For this review, take the finished solid that the model builds, in its own axes (mm). Give positions to 0.01 mm unless a question says otherwise; leave off trailing zeros. Write each loop counter-clockwise with the first axis right and the second up, starting at its lowest first coordinate (ties: lowest second). Pieces come first, ordered by that corner, then holes. Notation, with made-up numbers: (-25.75, 76) -> (-17.75, 76) arc R33 cw to (-17.75, 110) -> close; hole circle Ø8 at (86.5, 26.25). An arc over 180 degrees is marked (long way). Return JSON: item names as keys, results as strings.
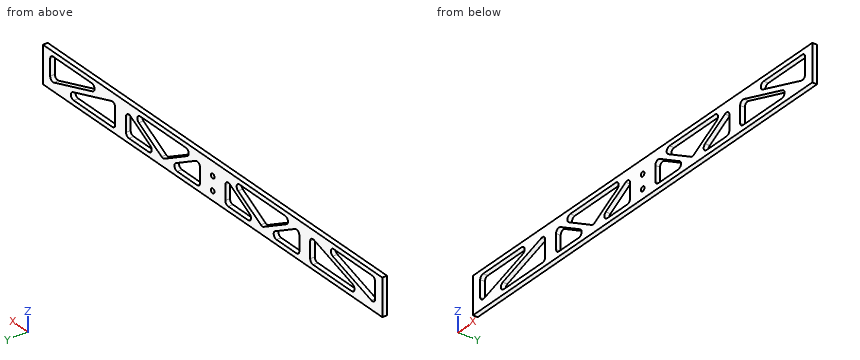
from build123d import *

# Parameters (mm, degrees)
SKETCH1_W           = 298.45
SKETCH1_H           = 25.4
BOSS_EXTRUDE1_DEPTH = 3.175
CUT_EXTRUDE1_DEPTH  = 4.175
SKETCH3_R           = 1.5875
CUT_EXTRUDE2_DEPTH  = 4.175
FILLET1_R           = 2.54


with BuildPart() as part:
    # Sketch1 → Boss-Extrude1 (new body)
    with BuildSketch(Plane(origin=(0, 0, 0), x_dir=(1, 0, 0), z_dir=(0, 1, 0))):
        Rectangle(SKETCH1_W, SKETCH1_H)
    extrude(amount=BOSS_EXTRUDE1_DEPTH)

    # Sketch2 → Cut-Extrude1 (cut, through all)
    with BuildSketch(Plane(origin=(0, 3.175, 0), x_dir=(1, 0, 0), z_dir=(0, 1, 0))):
        Polygon((-142.875, -9.525), (-90.745115786, -9.525), (-142.875, 7.851628071), align=None)
        Polygon((-85.725, -7.851628071), (-85.725, 9.525), (-137.854884214, 9.525), align=None)
        Polygon((-76.2, -7.685517516), (-46.798699244, 9.525), (-76.2, 9.525), align=None)
        Polygon((-73.057550756, -9.525), (-14.254949244, -9.525), (-43.65625, 7.685517516), align=None)
        Polygon((-11.1125, -7.685517516), (-11.1125, 9.525), (-40.513800756, 9.525), align=None)
        Polygon((11.1125, -7.685517516), (40.513800756, 9.525), (11.1125, 9.525), align=None)
        Polygon((14.254949244, -9.525), (73.057550756, -9.525), (43.65625, 7.685517516), align=None)
        Polygon((76.2, -7.685517516), (76.2, 9.525), (46.798699244, 9.525), align=None)
        Polygon((85.725, -7.851628071), (137.854884214, 9.525), (85.725, 9.525), align=None)
        Polygon((90.745115786, -9.525), (142.875, -9.525), (142.875, 7.851628071), align=None)
    extrude(amount=-CUT_EXTRUDE1_DEPTH, mode=Mode.SUBTRACT)

    # Sketch3 → Cut-Extrude2 (cut, through all)
    with BuildSketch(Plane(origin=(0, 3.175, 0), x_dir=(1, 0, 0), z_dir=(0, 1, 0))):
        with Locations((0, 6.35)):
            Circle(SKETCH3_R)
        with Locations((0, -3.175)):
            Circle(SKETCH3_R)
    extrude(amount=-CUT_EXTRUDE2_DEPTH, mode=Mode.SUBTRACT)

    # Fillet1
    fillet1_edges = [part.edges().sort_by_distance(p)[0] for p in [
        (-43.65625, 1.5875, -7.685517516),
        (-14.254949244, 1.5875, 9.525),
        (-73.057550756, 1.5875, 9.525),
        (-40.513800756, 1.5875, -9.525),
        (-11.1125, 1.5875, -9.525),
        (-11.1125, 1.5875, 7.685517516),
        (-76.2, 1.5875, 7.685517516),
        (-76.2, 1.5875, -9.525),
        (-46.798699244, 1.5875, -9.525),
        (-85.725, 1.5875, 7.851628071),
        (-137.854884214, 1.5875, -9.525),
        (-85.725, 1.5875, -9.525),
        (85.725, 1.5875, 7.851628071),
        (85.725, 1.5875, -9.525),
        (137.854884214, 1.5875, -9.525),
        (46.798699244, 1.5875, -9.525),
        (76.2, 1.5875, -9.525),
        (76.2, 1.5875, 7.685517516),
        (11.1125, 1.5875, 7.685517516),
        (11.1125, 1.5875, -9.525),
        (40.513800756, 1.5875, -9.525),
        (43.65625, 1.5875, -7.685517516),
        (73.057550756, 1.5875, 9.525),
        (14.254949244, 1.5875, 9.525),
        (90.745115786, 1.5875, 9.525),
        (142.875, 1.5875, -7.851628071),
        (142.875, 1.5875, 9.525),
        (-90.745115786, 1.5875, 9.525),
        (-142.875, 1.5875, 9.525),
        (-142.875, 1.5875, -7.851628071),
    ]]
    fillet(fillet1_edges, radius=FILLET1_R)


solid = part.part
1. For pin 1 (12 mm diameter, centred on x = 12, z = 7.5, fed in from -Y), flat-tipped, find the tip position at first contact; note if it passes through.
Results found:
{"pin 1": "stops at y = 0"}
2. To check wall thickness, follow probe 1 along Z at (x, y) = (0, 2.2); probe 2 along Z at (x, y) = (58, 1.65) (3 decimals); probe 3 along X at (y, z) = (1.95, 8.25) (3 decimals). State the ranges of each line that lie inside material, in increasing order.
Results found:
{"probe 1": "z = -12.7 to -7.94, -4.76 to 1.59, 4.76 to 12.7", "probe 2": "z = -12.7 to -9.525, -2.968 to 0.711, 9.525 to 12.7", "probe 3": "x = -149.225 to -142.538, -104.195 to -65.893, -21.419 to 21.419, 65.893 to 104.195, 142.538 to 149.225"}
3. Add section C-C, the plane x = 128.5. State the section outline as (y, z) points (3 decimals), plus the area to 3 significant figures.
Results found:
{"outline": "(0, -12.7) -> (3.175, -12.7) -> (3.175, -3.06) -> (0, -3.06) -> close; (0, 9.525) -> (3.175, 9.525) -> (3.175, 12.7) -> (0, 12.7) -> close", "area": "40.7 mm²"}
4. Add section A-A, the plane x = -39. State the section outline as (y, z) points (3 decimals), plus the area to 3 significant figures.
Results found:
{"outline": "(0, -12.7) -> (3.175, -12.7) -> (3.175, -4.96) -> (0, -4.96) -> close; (0, 9.525) -> (3.175, 9.525) -> (3.175, 12.7) -> (0, 12.7) -> close", "area": "34.7 mm²"}
5. Add section B-B, the plane y = 2.1. Count the separate pieces of the cut face and the enclosed holes in it, plus the area to 3 significant figures.
Results found:
{"separate pieces": "1", "enclosed holes": "12", "area": "4,020 mm²"}
